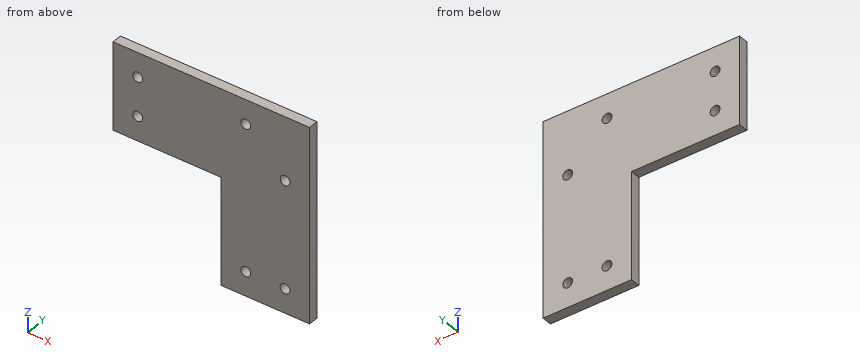
from build123d import *

# Parameters (mm, degrees)
SKETCH1_R           = 1.5875
BOSS_EXTRUDE1_DEPTH = 3.175


with BuildPart() as part:
    # Sketch1 → Boss-Extrude1 (new body)
    with BuildSketch(Plane(origin=(0, 0, 0), x_dir=(1, 0, 0), z_dir=(0, 1, 0))):
        Polygon((0, 0), (0, 28.575), (34.925, 28.575), (34.925, 63.5), (63.5, 63.5), (63.5, 0), align=None)
        with Locations(Location((7.9375, 20.6375, 0), (0, 0, 270))):
            Circle(SKETCH1_R, mode=Mode.SUBTRACT)
        with Locations(Location((7.9375, 7.9375, 0), (0, 0, 270))):
            Circle(SKETCH1_R, mode=Mode.SUBTRACT)
        with Locations(Location((42.8625, 7.9375, 0), (0, 0, 270))):
            Circle(SKETCH1_R, mode=Mode.SUBTRACT)
        with Locations(Location((55.5625, 20.6375, 0), (0, 0, 270))):
            Circle(SKETCH1_R, mode=Mode.SUBTRACT)
        with Locations(Location((55.5625, 55.5625, 0), (0, 0, 270))):
            Circle(SKETCH1_R, mode=Mode.SUBTRACT)
        with Locations(Location((42.8625, 55.5625, 0), (0, 0, 270))):
            Circle(SKETCH1_R, mode=Mode.SUBTRACT)
    extrude(amount=BOSS_EXTRUDE1_DEPTH)


solid = part.part
Can you work these out from the model? Positions are in its coordinate system, mm. Give positions to 0.01 mm unless a question says otherwise; leave off trailing zeros. Write each loop counter-clockwise with the first axis right and the second up, starting at its lowest first coordinate (ties: lowest second). Pieces come first, ordered by that corner, then holes. Notation, with made-up numbers: (86.5, 84) -> (132.5, 84) arc R11 cw to (132.5, 98) -> close; hole circle Ø9 at (81, -28). An arc over 180 degrees is marked (long way). Answer as a JSON object with one key per item and string values. Group by question number.
Item 1: Please list where these lines run through material, in increasing order: line 1 (Z direction, x = 8, y = 2) (3 decimals); line 2 (Z direction, x = 56, y = 1.05); line 3 (X direction, y = 2.4, z = -19.5). Write a range as [from, to].
Item 2: Suppose I cut it at D-D (x = 12.5). Please give me the cut outline in (y, z) (3 decimals), plus the area to 3 significant figures.
Item 3: Suppose I cut it at C-C (z = -33.5). Please give me the cut outline in (x, y) (3 decimals).
Item 4: Suppose I cut it at A-A (z = -8.5). Please give me the cut outline in (x, y) (3 decimals).
Item 5: Suppose I cut it at B-B (y = 1.5). State how many separate pieces and enclosed holes the cut face has, plus the area to 3 significant figures.
Item 6: I'm going to push flat-ended pins straight in: P1, Ø3, axis at x = 7.94, z = -20.64, coming from the -Y side; P2, Ø5, axis at x = 42.86, z = -7.94, coming from the -Y side; P3, Ø1, axis at y = 2, z = -45.5, coming from the -X side (3 decimals); P4, Ø1, axis at x = 19, y = 1, coming from the -Z side (3 decimals). Where does each tip first touch, or does it pass through?
Findings:
{
 "1": {"line 1": "z = [-28.575, -22.224], [-19.051, -9.524], [-6.351, 0]", "line 2": "z = [-63.5, -57.09], [-54.04, -22.16], [-19.11, 0]", "line 3": "x = [0, 6.83], [9.04, 54.46], [56.67, 63.5]"},
 "2": {"outline": "(0, -28.575) -> (3.175, -28.575) -> (3.175, 0) -> (0, 0) -> close", "area": "90.7 mm²"},
 "3": {"outline": "(34.925, 0) -> (63.5, 0) -> (63.5, 3.175) -> (34.925, 3.175) -> close"},
 "4": {"outline": "(0, 0) -> (6.453, 0) -> (6.453, 3.175) -> (0, 3.175) -> close; (9.422, 0) -> (41.378, 0) -> (41.378, 3.175) -> (9.422, 3.175) -> close; (44.347, 0) -> (63.5, 0) -> (63.5, 3.175) -> (44.347, 3.175) -> close"},
 "5": {"separate pieces": "1", "enclosed holes": "6", "area": "2,760 mm²"},
 "6": {"P1": "passes through", "P2": "stops at y = 0", "P3": "stops at x = 34.925", "P4": "stops at z = -28.575"}
}
